The listing builds one solid part. Answer for the finished solid, in the listing's coordinates (mm). Face numbers are marked on the shaded views. A direction names the side the tool comes from. Round coordinates to 2 decimals unless told otherwise and drop trailing zeros. Write each loop counter-clockwise with the first axis right and the second up, starting at its lowest first coordinate (ties: lowest second). Pieces come first, ordered by that corner, then holes. Notation, with made-up numbers: (27.25, 49) - (44.25, 49) arc R36 cw to (44.25, 85) - close; hole circle Ø4 at (-27.5, 5.25). An arc over 180 degrees is marked (long way). Use a Markdown table: item, result. Add a question column.
1) Determine the mould class of the marked faces 1, 2 and 3 for opening direction Y: +Y half, -Y half, draft (parallel to the pull), parting line (faces both ways), or undercut.
2) A cutting plane is placed at B-B (x = -0.5). Give the vertices of the cut face in (y, z).
3) Each of these flat-tipped pins is pushed along its axis until it touches: P1, Ø2, axis at x = 3, z = -5.5, coming from the +Y side; P2, Ø0.8, axis at x = 6.5, y = 3.5, coming from the -Z side; P3, Ø1, axis at y = 3.5, z = 6.5, coming from the +X side. Where does it stop, or does it pass through?
4) A cutting plane is placed at D-D (z = 2). Give the vertices of the cut face in (x, y).
5) Find the intervals of material crossed by probe 1 along Y at (x, z) = (-0.75, 5); probe 2 along X at (y, z) = (2.75, 4.75); probe 3 along X at (y, z) = (3.4, -3.25), in increasing order. Write a range as from..to.
6) A cutting plane is placed at C-C (z = -6). Give the vertices of the cut face in (x, y).
7) A cutting plane is placed at A-A (y = 3.65). Give the vertices of the cut face in (x, z), then the cut area to 3 significant figures.
8) A tool of negligible diameter and unlimited length cuts with its end or side. For the marked faces 4, 5 and 6, from which of +Z, -Z, +X, -X, +Y, -Y can it reach the whole face along a straight path? Write none if from no direction.
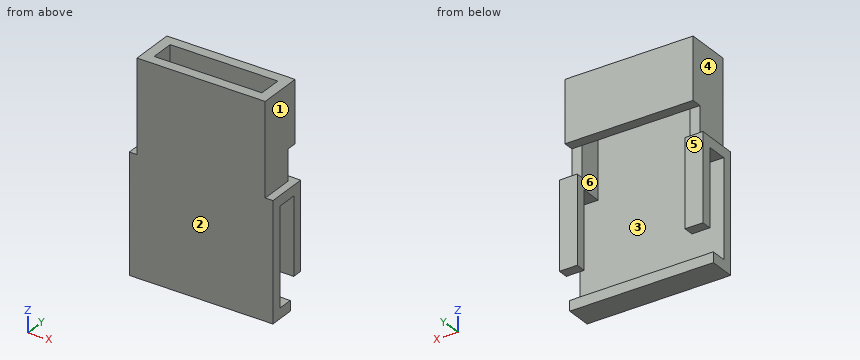
```python
from build123d import *

# Parameters (mm, degrees)
SKETCH_2_W           = 12
SKETCH_2_H           = 9.5
SKETCH_2_W_2         = 10.5
SKETCH_2_H_2         = 9
EXTRUDE_1_DEPTH      = 1
EXTRUDE_2_DEPTH      = 2.3
EXTRUDE_2_DEPTH_BACK = 1
SKETCH_4_W           = 1
SKETCH_4_H           = 9.5
SKETCH_4_W_2         = 10.5
SKETCH_4_H_2         = 1
CUT_EXTRUDE_1_DEPTH  = 2.3
SKETCH_5_W           = 12.5
SKETCH_5_H           = 6
EXTRUDE_3_DEPTH      = 1
SKETCH_6_W           = 1.75
SKETCH_6_H           = 1
CUT_EXTRUDE_3_DEPTH  = 0.3
SKETCH_9_W           = 14
SKETCH_9_H           = 1
CUT_EXTRUDE_4_DEPTH  = 0.8
SKETCH_10_W          = 1.75
SKETCH_10_H          = 7.5
SKETCH_10_H_2        = 8.5
EXTRUDE_7_DEPTH      = 1


with BuildPart() as part:
    # 草图2 → 凸台-拉伸1 (new body)
    with BuildSketch(Plane(origin=(0, 0, 0), x_dir=(1, 0, 0), z_dir=(0, 1, 0))):
        with Locations((0, 4.75)):
            Rectangle(SKETCH_2_W, SKETCH_2_H)
        with Locations((0, -4.5)):
            Rectangle(SKETCH_2_W_2, SKETCH_2_H_2)
    extrude(amount=EXTRUDE_1_DEPTH)

    # 草图3 → 凸台-拉伸2 (add, two sides)
    with BuildSketch(Plane(origin=(0, 1, 0), x_dir=(1, 0, 0), z_dir=(0, 1, 0))) as extrude_2_sk:
        Polygon((7, -1), (7, 10.5), (-7, 10.5), (-7, -1), (-6.25, -1), (-6.25, -10), (6.25, -10), (6.25, -1), align=None)
        Polygon((6, 0), (6, 9.5), (-6, 9.5), (-6, 0), (-5.25, 0), (-5.25, -9), (5.25, -9), (5.25, 0), align=None, mode=Mode.SUBTRACT)
    extrude(amount=EXTRUDE_2_DEPTH)
    extrude(extrude_2_sk.sketch, amount=-EXTRUDE_2_DEPTH_BACK)

    # 草图4 → 切除-拉伸1 (cut)
    with BuildSketch(Plane(origin=(0, 3.3, 0), x_dir=(1, 0, 0), z_dir=(0, 1, 0))):
        with Locations((-6.5, 4.75)):
            Rectangle(SKETCH_4_W, SKETCH_4_H)
        with Locations((6.5, 4.75)):
            Rectangle(SKETCH_4_W, SKETCH_4_H)
        with Locations((0, -9.5)):
            Rectangle(SKETCH_4_W_2, SKETCH_4_H_2)
    extrude(amount=-CUT_EXTRUDE_1_DEPTH, mode=Mode.SUBTRACT)

    # 草图5 → 凸台-拉伸3 (add)
    with BuildSketch(Plane(origin=(0, 3.3, 0), x_dir=(1, 0, 0), z_dir=(0, 1, 0))):
        with Locations((0, -7)):
            Rectangle(SKETCH_5_W, SKETCH_5_H)
    extrude(amount=EXTRUDE_3_DEPTH)

    # 草图6 → 切除-拉伸3 (cut)
    with BuildSketch(Plane(origin=(0, 3.3, 0), x_dir=(1, 0, 0), z_dir=(0, 1, 0))):
        with Locations((-6.125, -0.5)):
            Rectangle(SKETCH_6_W, SKETCH_6_H)
        with Locations((6.125, -0.5)):
            Rectangle(SKETCH_6_W, SKETCH_6_H)
    extrude(amount=-CUT_EXTRUDE_3_DEPTH, mode=Mode.SUBTRACT)

    # 草图9 → 切除-拉伸4 (cut)
    with BuildSketch(Plane(origin=(0, 3.3, 0), x_dir=(1, 0, 0), z_dir=(0, 1, 0))):
        with Locations((0, 10)):
            Rectangle(SKETCH_9_W, SKETCH_9_H)
    extrude(amount=-CUT_EXTRUDE_4_DEPTH, mode=Mode.SUBTRACT)

    # 草图10 → 凸台-拉伸7 (add)
    with BuildSketch(Plane(origin=(0, 3, 0), x_dir=(1, 0, 0), z_dir=(0, 1, 0))):
        with Locations((-6.125, 3.75)):
            Rectangle(SKETCH_10_W, SKETCH_10_H)
        with Locations((6.125, 3.25)):
            Rectangle(SKETCH_10_W, SKETCH_10_H_2)
        Polygon((-5.25, 0), (-7, 0), (-7, -1), (-6.25, -1), (-5.25, -1), align=None)
    extrude(amount=EXTRUDE_7_DEPTH)


solid = part.part
```
Entries:
| question | item | result |
|---|---|---|
| 1 | face 1 | draft |
| 1 | face 2 | -Y half |
| 1 | face 3 | undercut |
| 2 | outline | (0, -10.5) - (2.5, -10.5) - (2.5, -9.5) - (1, -9.5) - (1, 10) - (0, 10) - close; (3.3, 4) - (4.3, 4) - (4.3, 10) - (3.3, 10) - close |
| 3 | P1 | stops at y = 1 |
| 3 | P2 | stops at z = -7.5 |
| 3 | P3 | stops at x = 6.25 |
| 4 | outline | (-6.25, 0) - (6.25, 0) - (6.25, 3.3) - (5.25, 3.3) - (5.25, 1) - (-5.25, 1) - (-5.25, 3.3) - (-6.25, 3.3) - close |
| 5 | probe 1 | y = 0..1, 3.3..4.3 |
| 5 | probe 2 | x = -6.25..-5.25, 5.25..6.25 |
| 5 | probe 3 | x = -7..-5.25, 5.25..7 |
| 6 | outline | (-7, 0) - (7, 0) - (7, 1) - (-7, 1) - close; (-7, 3) - (-5.25, 3) - (-5.25, 4) - (-7, 4) - close; (5.25, 3) - (7, 3) - (7, 4) - (5.25, 4) - close |
| 7 | outline | (-7, -7.5) - (-5.25, -7.5) - (-5.25, 1) - (-7, 1) - close; (-6.25, 4) - (6.25, 4) - (6.25, 10) - (-6.25, 10) - close; (5.25, -7.5) - (7, -7.5) - (7, 1) - (5.25, 1) - close |
| 7 | area | 105 mm² |
| 8 | face 4 | +Z, -X, +Y, -Y |
| 8 | face 5 | -Z, +X, -X, +Y |
| 8 | face 6 | none |
